Input: dimensioned drawing with shaded views. Units: mm. Origin: part minimum x, y, z. A direction names the side the tool comes from. Give positions to 0.01 mm unless a question says otherwise; leave off trailing zeros. Loops run counter-clockwise (first coordinate to the right, second up) from the corner with the lowest first, then second, coordinate; pieces in that order, holes last.
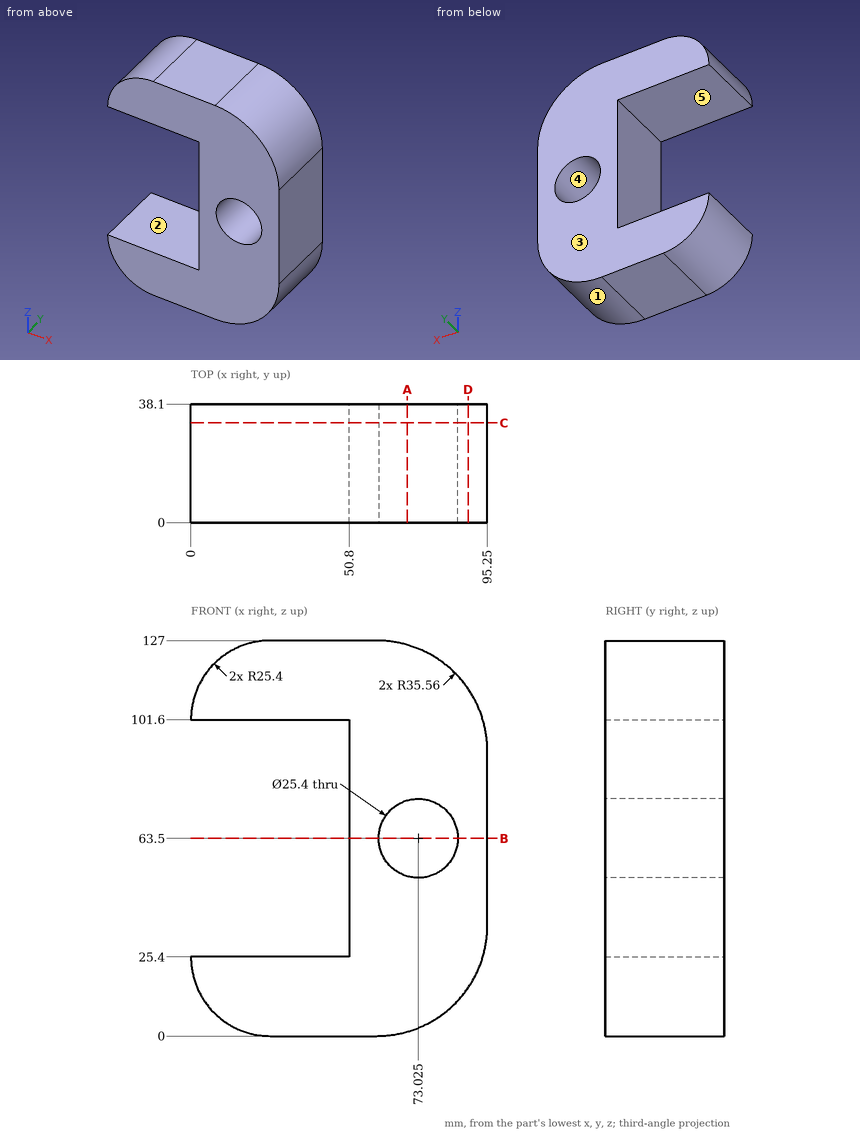
Item 1: Section query B-B on z = 63.5. Return loops of the section in (x, y) (3 decimals), plus the area to 3 significant figures.
Values follow:
outline: (50.8, 0) - (60.325, 0) - (60.325, 38.1) - (50.8, 38.1) - close; (85.725, 0) - (95.25, 0) - (95.25, 38.1) - (85.725, 38.1) - close
area: 726 mm2
Item 2: Ray query, probe 1 along Z at (x, y) = (36.5, 12.5); probe 2 along X at (y, z) = (29, 63); probe 3 along X at (y, z) = (4, 86). Return the intervals inside material, ascending.
Values follow:
probe 1: z = 0 to 25.4, 101.6 to 127
probe 2: x = 50.8 to 60.33, 85.72 to 95.25
probe 3: x = 50.8 to 95.25
Item 3: Pin query (flat end, axial travel): pin 1 (12 mm diameter, centred on x = 64, y = 16, fed in from +Z); pin 2 (4 mm diameter, centred on x = 18, y = 33.5, fed in from +Z); pin 3 (12 mm diameter, centred on y = 32, z = 80, fed in from -X); pin 4 (2 mm diameter, centred on x = 48.5, z = 40.5, fed in from -Y). Return the tip coordinate at first contact, or that it passes through.
Values follow:
pin 1: stops at z = 127
pin 2: stops at z = 126.42
pin 3: stops at x = 50.8
pin 4: passes through
Item 4: Draft query along Z for the marked faces 1, 2 and 3. Return one class per face: +Z half, -Z half, draft (parallel to the pull), parting line (faces both ways), or undercut.
Values follow:
face 1: -Z half
face 2: undercut
face 3: draft
Item 5: Set-up query: the marked faces 4 and 5. Return all of +Z, -Z, +X, -X, +Y, -Y with unobstructed straight access to the full face (end or side cutting, diameter ignored); none if empty.
Values follow:
face 4: +Y, -Y
face 5: -X, +Y, -Y
Item 6: Section query D-D on x = 89. Return loops of the section in (y, z), plus the area to 3 significant figures.
Values follow:
outline: (0, 15.42) - (38.1, 15.42) - (38.1, 111.58) - (0, 111.58) - close
area: 3,660 mm2
Item 7: Section query A-A on x = 69.5. Return loops of the section in (y, z), plus the area to 3 significant figures.
Values follow:
outline: (0, 1.38) - (38.1, 1.38) - (38.1, 51.3) - (0, 51.3) - close; (0, 75.7) - (38.1, 75.7) - (38.1, 125.62) - (0, 125.62) - close
area: 3,800 mm2
Item 8: Section query C-C on y = 32. Return loops of the section in (x, z) (3 decimals), plus the area to 3 significant figures.
Values follow:
outline: (0, 25.4) arc R25.4 ccw to (25.4, 0) - (59.69, 0) arc R35.56 ccw to (95.25, 35.56) - (95.25, 91.44) arc R35.56 ccw to (59.69, 127) - (25.4, 127) arc R25.4 ccw to (0, 101.6) - (50.8, 101.6) - (50.8, 25.4) - close; hole circle Ø25.4 at (73.025, 63.5)
area: 6,900 mm2
